Study the drawing (mm; zero at the part's minimum x, y, z) and answer. A direction names the side the tool comes from. Round coordinates to 2 decimals unless told otherwise and drop trailing zeros. Write each loop counter-clockwise with the first axis right and the second up, starting at its lowest first coordinate (ties: lowest second). Pieces come first, ordered by that corner, then holes. Notation, with made-up numbers: (-6, -33.5) - (35, -33.5) arc R15 ccw to (35, -7.5) - close; hole circle Ø1 at (65, 21). An arc over 180 degrees is marked (long way). Return JSON: item names as keys, results as strings. Group by question number.
(1) Section A-A, the plane y = 3.75 is taken. Write down the section's boundary in (x, z), then the cut area to 3 significant figures.
(2) Section D-D, the plane y = 6.5 is taken. Write down the section's boundary in (x, z).
(3) Find the intervals of material crossed by line 1 along X through (y, z) = (5.25, 1.4); line 2 along X through (y, z) = (5.75, 2.55); line 3 along X through (y, z) = (6.5, 2.7), in increasing order. Write a range as [from, to].
(4) Determine the mould class of the marked faces 6, 7, 8 and 9 for opening direction X: +X half, -X half, draft (parallel to the pull), parting line (faces both ways), or undercut.
(5) Which of the six approach directions +Z, -Z, +X, -X, +Y, -Y give full straight-line access (tool end or side, diameter ignored) to the marked faces 1, 2, 3, 4 and 5?
(6) Section B-B, the plane z = 0.75 is taken. Write down the section's boundary in (x, y) (3 decimals).
(7) Section C-C, the plane x = 11.25 is taken. Write down the section's boundary in (y, z), then the cut area to 3 significant figures.
(8) This flat-tipped pin is pushed along its axis until it touches: pin 1 (0.9 mm diameter, centred on x = 4.5, z = 1.5, fed in from +Y). Where does it stop, or does it pass through?
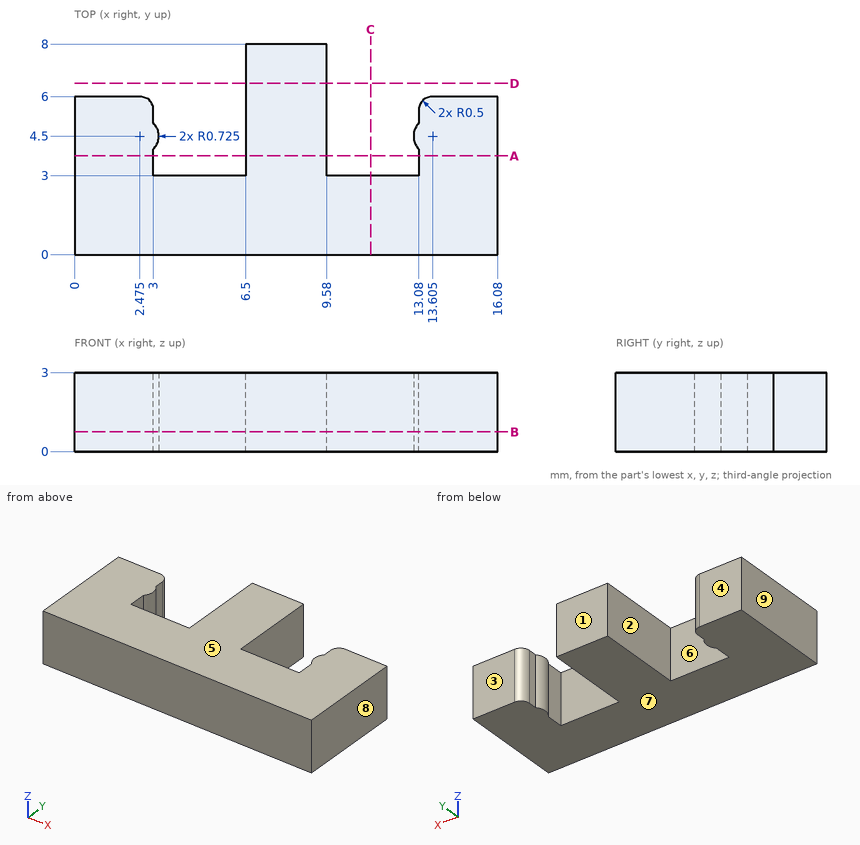
Working result:
{
 "1": {"outline": "(0, 0) - (3, 0) - (3, 3) - (0, 3) - close; (6.5, 0) - (9.58, 0) - (9.58, 3) - (6.5, 3) - close; (13.08, 0) - (16.08, 0) - (16.08, 3) - (13.08, 3) - close", "area": "27.2 mm^2"},
 "2": {"outline": "(6.5, 0) - (9.58, 0) - (9.58, 3) - (6.5, 3) - close"},
 "3": {"line 1": "x = [0, 3], [6.5, 9.58], [13.08, 16.08]", "line 2": "x = [0, 2.93], [6.5, 9.58], [13.15, 16.08]", "line 3": "x = [6.5, 9.58]"},
 "4": {"face 6": "undercut", "face 7": "draft", "face 8": "+X half", "face 9": "-X half"},
 "5": {"face 1": "+Z, -Z, +X, -X, +Y", "face 2": "+Z, -Z, +Y", "face 3": "+Z, -Z, +X, +Y", "face 4": "+Z, -Z, -X, +Y", "face 5": "+Z, +X, -X, +Y, -Y"},
 "6": {"outline": "(0, 0) - (16.08, 0) - (16.08, 6) - (13.58, 6) arc R0.5 ccw to (13.08, 5.5) - (13.08, 5) arc R0.725 ccw to (13.08, 4) - (13.08, 3) - (9.58, 3) - (9.58, 8) - (6.5, 8) - (6.5, 3) - (3, 3) - (3, 4) arc R0.725 ccw to (3, 5) - (3, 5.5) arc R0.5 ccw to (2.5, 6) - (0, 6) - close"},
 "7": {"outline": "(0, 0) - (3, 0) - (3, 3) - (0, 3) - close", "area": "9.00 mm^2"},
 "8": {"pin 1": "stops at y = 3"}
}
